from build123d import *

# Parameters (mm, degrees)
BOSS_EXTRUDE1_DEPTH  = 75
FILLET1_R            = 6.35
SKETCH2_R            = 21
CUT_EXTRUDE1_DEPTH   = 75
CIRPATTERN1_COUNT    = 4
M6_CLEARANCE_HOLE1_D = 6.4


with BuildPart() as part:
    # Sketch1 → Boss-Extrude1 (new body)
    with BuildSketch(Plane(origin=(0, 0, 0), x_dir=(0, 0, -1), z_dir=(1, 0, 0))):
        with BuildLine():
            Line((0, 0), (0, 101.6))
            Line((0, 101.6), (6.35, 101.6))
            Line((6.35, 101.6), (6.35, 15.875))
            ThreePointArc((6.35, 15.875), (9.139807909, 9.139807909), (15.875, 6.35))
            Line((15.875, 6.35), (101.6, 6.35))
            Line((101.6, 6.35), (101.6, 0))
            Line((101.6, 0), (0, 0))
        make_face()
    extrude(amount=BOSS_EXTRUDE1_DEPTH)

    # Fillet1
    fillet1_edges = [part.edges().sort_by_distance(p)[0] for p in [
        (37.5, 0, 0),
    ]]
    fillet(fillet1_edges, radius=FILLET1_R)

    # Sketch2 → Cut-Extrude1 (cut)
    with BuildSketch(Plane(origin=(0, 0, 0), x_dir=(-1, 0, 0), z_dir=(0, 0, -1))):
        with Locations((-37.5, 70)):
            Circle(SKETCH2_R)
    extrude(amount=CUT_EXTRUDE1_DEPTH, mode=Mode.SUBTRACT)

    # Sketch13 → CSK for M5 Flat Head Machine Screw3 (revolve, cut)
    with BuildSketch(Plane(origin=(55.884776311, 88.384776311, 0), x_dir=(0, -1, 0), z_dir=(1, 0, 0))):
        Polygon((0, 0), (0, 14.29228064), (2.65, 12.7), (2.65, 2.55), (5.2, 0), align=None)
    csk_for_m5_flat_head_machine_screw3 = revolve(axis=Axis((55.884776311, 88.384776311, 6.35), (0, 0, -1)), mode=Mode.SUBTRACT)

    # CirPattern1: CSK for M5 Flat Head Machine Screw3 ×4 about axis
    cirpattern1_axis = Axis((37.5, 70, 0), (0, 0, 1))
    for i in range(1, CIRPATTERN1_COUNT):
        add(csk_for_m5_flat_head_machine_screw3.rotate(cirpattern1_axis, i * 360 / CIRPATTERN1_COUNT), mode=Mode.SUBTRACT)

    # M6 Clearance Hole1 (through all)
    with Locations(Plane(origin=(37.5, 6.35, -85.729264805), x_dir=(0, 0, 1), z_dir=(0, 1, 0))):
        with Locations((0, 0), (47.631397208, 27.5), (47.631397208, -27.5)):
            Hole(M6_CLEARANCE_HOLE1_D / 2)


solid = part.part
Check sheet for the modelled part. Datum: model origin and axes. Units: mm. A direction names the side the tool comes from. Give positions to 0.01 mm unless a question says otherwise; leave off trailing zeros. Order: outer loops, then holes, each group sorted by start corner. A loop starts at its lowest first (then second) coordinate and runs counter-clockwise, first axis right, second up. Notation, with made-up numbers: (-6, -9) - (39, -9) arc R12 cw to (39, -1) - close; hole circle Ø10 at (20, -3). An arc over 180 degrees is marked (long way). Answer as CSV lines item,"result".
1. Tool access check on faces 4 (the face through (38.02, 1.91, -1.81)), 5 (the face through (45, 50, -6.35)). Record the directions out of +Z, -Z, +X, -X, +Y, -Y that give a thin tool (end or side, any length) a straight path to the whole face; none if there is none.
Result sheet:
face 4,"+Z, +X, -X, -Y"
face 5,"-Z, +X, -X, +Y"
2. Section check C-C (y = 70). Record the boundary of the cut face in (x, z).
Result sheet:
outline,"(0, -6.35) - (16.5, -6.35) - (16.5, 0) - (0, 0) - close; (58.5, -6.35) - (75, -6.35) - (75, 0) - (58.5, 0) - close"
3. Scan lines: probe 1 along Y at (x, z) = (24, -81.5); probe 2 along Z at (x, y) = (7, 47); probe 3 along Y at (x, z) = (37.5, -1.75). Record each from-to range of solid material in increasing order. Write a range as from..to.
Result sheet:
probe 1,"0..6.35"
probe 2,"-6.35..0"
probe 3,"1.97..49, 91..101.6"
4. Mould release check, pull along X, two halves, no side actions. Record for faces 1 (the face through (61.876, 3.131, -37.404)), 2 (the face through (0, 6, -28)), 3 (the face through (37, 6.35, -58)): released by +X, released by -X, zero draft, split by the parting line, or undercut.
Result sheet:
face 1,"undercut"
face 2,"released by -X"
face 3,"zero draft"
5. Section check A-A (x = 10). Record the boundary of the cut face in (y, z) (3 decimals).
Result sheet:
outline,"(0, -101.6) - (6.35, -101.6) - (6.35, -41.298) - (0, -41.298) - close; (0, -34.898) - (6.35, -34.898) - (6.35, -15.875) arc R9.525 cw to (15.875, -6.35) - (101.6, -6.35) - (101.6, 0) - (6.35, 0) arc R6.35 ccw to (0, -6.35) - close"
6. Section check D-D (z = -19). Record the boundary of the cut face in (x, y).
Result sheet:
outline,"(0, 0) - (75, 0) - (75, 6.35) - (0, 6.35) - close"
7. Section check B-B (x = 37.5). Record the boundary of the cut face in (y, z) (3 decimals).
Result sheet:
outline,"(0, -101.6) - (6.35, -101.6) - (6.35, -88.929) - (0, -88.929) - close; (0, -82.529) - (6.35, -82.529) - (6.35, -15.875) arc R9.525 cw to (15.875, -6.35) - (49, -6.35) - (49, 0) - (6.35, 0) arc R6.35 ccw to (0, -6.35) - close; (91, -6.35) - (101.6, -6.35) - (101.6, 0) - (91, 0) - close"
8. Go/stop test with flat-tipped pins: P1, Ø4, axis at x = 10, z = -38.1, coming from the +Y side; P2, Ø8.5, axis at x = 19.12, y = 88.38, coming from the +Z side; P3, Ø2, axis at x = 62.5, z = -30, coming from the +Y side. Record where each tip stops, or that it passes through.
Result sheet:
P1,"through"
P2,"z = -0.94"
P3,"y = 6.35"
